from build123d import *

# Parameters (mm, degrees)
BOSS_EXTRUDE4_DEPTH = 15
SKETCH3_R           = 7.86
BOSS_EXTRUDE2_DEPTH = 3
BOSS_EXTRUDE3_DEPTH = 7.32
SKETCH6_R           = 0.715
CUT_EXTRUDE2_DEPTH  = 17.35
FILLET5_R           = 0.8


with BuildPart() as part:
    # Sketch8 → Boss-Extrude4 (new body, symmetric)
    with BuildSketch(Plane(origin=(0, 0, 0), x_dir=(0, 0, -1), z_dir=(1, 0, 0))):
        Polygon((-9, 0), (9, 10.392304845), (9, 0), align=None)
    extrude(amount=BOSS_EXTRUDE4_DEPTH, both=True)

    # Sketch3 → Boss-Extrude2 (add)
    with BuildSketch(Plane(origin=(0, 1.640246968, 6.159008915), x_dir=(1, 0, 0), z_dir=(0, -0.866025404, -0.5))):
        with Locations((0, -7.11181091)):
            Circle(SKETCH3_R)
    extrude(amount=-BOSS_EXTRUDE2_DEPTH)

    # Sketch5 → Boss-Extrude3 (add)
    with BuildSketch(Plane(origin=(0, 6.495190528, 3.75), x_dir=(1, 0, 0), z_dir=(0, 0.866025404, 0.5))):
        with BuildLine():
            Line((1.35, 4.588434219), (1.35, 5.674941499))
            ThreePointArc((1.35, 5.674941499), (0, 5.958076211), (-1.35, 5.674941499))
            Line((-1.35, 5.674941499), (-1.35, 4.588434219))
            ThreePointArc((-1.35, 4.588434219), (-2.405, 2.598076211), (-1.35, 0.607718203))
            Line((-1.35, 0.607718203), (-1.35, -0.478789077))
            ThreePointArc((-1.35, -0.478789077), (0, -0.761923789), (1.35, -0.478789077))
            Line((1.35, -0.478789077), (1.35, 0.607718203))
            ThreePointArc((1.35, 0.607718203), (2.405, 2.598076211), (1.35, 4.588434219))
        make_face()
    extrude(amount=BOSS_EXTRUDE3_DEPTH)

    # Sketch6 → Cut-Extrude2 (cut, through all)
    with BuildSketch(Plane(origin=(1.35, 0, 0), x_dir=(0, 0, -1), z_dir=(1, 0, 0))):
        with Locations((-1.275154643, 14.124785052)):
            Circle(SKETCH6_R)
        with Locations((-7.094845357, 10.764785052)):
            Circle(SKETCH6_R)
    extrude(amount=-CUT_EXTRUDE2_DEPTH, mode=Mode.SUBTRACT)

    # Fillet5
    fillet5_edges = [part.edges().sort_by_distance(p)[0] for p in [
        (0, 12.45353459, 8.069845357),
        (0, 15.81353459, 2.250154643),
    ]]
    fillet(fillet5_edges, radius=FILLET5_R)


solid = part.part
Source: CAD feature listing. Evaluate the final solid. Frame: model axes, mm. A direction names the side the tool comes from. Coordinates: 2 decimals unless noted, no trailing zeros. Loops run counter-clockwise (first coordinate to the right, second up) from the corner with the lowest first, then second, coordinate; pieces in that order, holes last. Notation, with made-up numbers: (-15, 47.5) -> (18, 47.5) arc R23 cw to (18, 78.5) -> close; hole circle Ø2 at (19, -13.5). An arc over 180 degrees is marked (long way). Answer in a Markdown table with one row per item. Add a question column.
Q1. Section A-A on x = 4.5. Return the cut outline in (y, z).
Q2. Ray query, line 1 along Z through (x, y) = (-0.25, 10.25); line 2 along Z through (x, y) = (10.75, 3.5); line 3 along Y through (x, z) = (-1.5, 4.5). Return the intervals inside material, ascending.
Q3. Reachability of faces 5 (the face through (-1.35, 9.7, 5.5)), 6 (the face through (-1.857, 6.866, 3.108)), 7 (the face through (-1.35, 12, 1)) from +Z, -Z, +X, -X, +Y, -Y: full face, straight path, thin tool, end or side. Return the list, or none.
Q4. Contact query for flat-ended pins moving along their axis: pin 1 Ø2.5 at (y, z) = (10.5, 1.5) entering from +X; pin 2 Ø1.3 at (y, z) = (8.5, 5.5) entering from -X; pin 3 Ø3 at (x, y) = (4, 11.5) entering from -Z. Output: stop coordinate, or through.
Q5. Section B-B on x = -7.25. Return the cut outline in (y, z), and give its area (3 significant figures).
Q6. Pull-direction query (Y, two-part tool) for faces 1 (the face through (0, 0, 0)), 2 (the face through (0.02, 13.78, 1.9)), 3 (the face through (0.019, 11.487, -0.248)), 4 (the face through (1.35, 12, 1)); classes: pulls with the +Y half, pulls with the -Y half, needs draft (parallel to the pull), parting line crosses it, or undercut.
Computed values:
| question | item | result |
|---|---|---|
| 1 | outline | (0, -9) -> (10.39, -9) -> (8.42, -5.58) -> (11.02, -4.08) -> (4.57, 7.08) -> (1.97, 5.58) -> (0, 9) -> close |
| 2 | line 1 | z = -9 to -8.75, -6.15 to -2.75, -0.95 to 6.6 |
| 2 | line 2 | z = -9 to 2.94 |
| 2 | line 3 | y = 0 to 6.06, 9.23 to 14.51 |
| 3 | face 5 | +Z, -X |
| 3 | face 6 | none |
| 3 | face 7 | -X, +Y |
| 4 | pin 1 | stops at x = 2.4 |
| 4 | pin 2 | stops at x = -1.35 |
| 4 | pin 3 | stops at z = -9 |
| 5 | outline | (0, -9) -> (10.39, -9) -> (6.71, -2.63) -> (9.31, -1.13) -> (6.28, 4.13) -> (3.68, 2.63) -> (0, 9) -> close |
| 5 | area | 112 mm^2 |
| 6 | face 1 | pulls with the -Y half |
| 6 | face 2 | undercut |
| 6 | face 3 | pulls with the +Y half |
| 6 | face 4 | needs draft |
